The listing builds one solid part. Answer for the finished solid, in the listing's coordinates (mm). A direction names the side the tool comes from. Give positions to 0.01 mm unless a question says otherwise; leave off trailing zeros. Write each loop counter-clockwise with the first axis right and the second up, starting at its lowest first coordinate (ties: lowest second). Pieces come first, ordered by that corner, then holes.
```python
from build123d import *

# Parameters (mm, degrees)
BOSS_EXTRUDE1_DEPTH = 57
SKETCH3_R           = 47.5
SKETCH3_R_2         = 31
BOSS_EXTRUDE3_DEPTH = 13
SKETCH4_R           = 47.5
SKETCH4_R_2         = 32.5
BOSS_EXTRUDE4_DEPTH = 37
SKETCH5_R           = 47.5
SKETCH5_R_2         = 31
BOSS_EXTRUDE5_DEPTH = 11
SKETCH8_R           = 19
BOSS_EXTRUDE6_DEPTH = 3
SKETCH9_W           = 85.5
SKETCH9_H           = 94
CUT_EXTRUDE1_DEPTH  = 3
CUT_EXTRUDE3_DEPTH  = 29.5
CUT_EXTRUDE4_DEPTH  = 36


with BuildPart() as part:
    # Sketch1 → Boss-Extrude1 (new body, symmetric)
    with BuildSketch(Plane(origin=(0, 0, 0), x_dir=(1, 0, 0), z_dir=(0, 1, 0))):
        Polygon((-102, 0), (-97, 16), (97, 16), (102, 0), (0, 0), align=None)
    extrude(amount=BOSS_EXTRUDE1_DEPTH, both=True)

    # Sketch3 → Boss-Extrude3 (add)
    with BuildSketch(Plane(origin=(0, 0, -16), x_dir=(-1, 0, 0), z_dir=(0, 0, -1))):
        with Locations(Location((0, 0, 0), (0, 0, 180))):  # turned: the seam where the file's is
            Circle(SKETCH3_R)
        Circle(SKETCH3_R_2, mode=Mode.SUBTRACT)
    extrude(amount=BOSS_EXTRUDE3_DEPTH)

    # Sketch4 → Boss-Extrude4 (add)
    with BuildSketch(Plane(origin=(0, 0, -29), x_dir=(-1, 0, 0), z_dir=(0, 0, -1))):
        with Locations(Location((0, 0, 0), (0, 0, 180))):  # turned: the seam where the file's is
            Circle(SKETCH4_R)
        Circle(SKETCH4_R_2, mode=Mode.SUBTRACT)
    extrude(amount=BOSS_EXTRUDE4_DEPTH)

    # Sketch5 → Boss-Extrude5 (add)
    with BuildSketch(Plane(origin=(0, 0, -66), x_dir=(-1, 0, 0), z_dir=(0, 0, -1))):
        with Locations(Location((0, 0, 0), (0, 0, 180))):  # turned: the seam where the file's is
            Circle(SKETCH5_R)
        Circle(SKETCH5_R_2, mode=Mode.SUBTRACT)
    extrude(amount=BOSS_EXTRUDE5_DEPTH)

    # Sketch8 → Boss-Extrude6 (add)
    with BuildSketch(Plane(origin=(0, 0, -16), x_dir=(-1, 0, 0), z_dir=(0, 0, -1))):
        with Locations(Location((-70, 28, 0), (0, 0, 180))):  # turned: the seam where the file's is
            Circle(SKETCH8_R)
        with Locations(Location((-70, -28, 0), (0, 0, 180))):  # turned: the seam where the file's is
            Circle(SKETCH8_R)
    boss_extrude6 = extrude(amount=BOSS_EXTRUDE6_DEPTH)

    # Sketch9 → Cut-Extrude1 (cut)
    with BuildSketch(Plane.XY):
        with Locations((49.25, 0)):
            Rectangle(SKETCH9_W, SKETCH9_H)
    cut_extrude1 = extrude(amount=-CUT_EXTRUDE1_DEPTH, mode=Mode.SUBTRACT)

    # Sketch6 → Cut-Extrude3 (cut, symmetric)
    with BuildSketch(Plane(origin=(0, 0, -16), x_dir=(-1, 0, 0), z_dir=(0, 0, -1))):
        with BuildLine():
            Line((-73, 36), (-67, 36))
            ThreePointArc((-67, 36), (-59, 28), (-67, 20))
            Line((-67, 20), (-73, 20))
            ThreePointArc((-73, 20), (-81, 28), (-73, 36))
        make_face()
    cut_extrude3 = extrude(amount=CUT_EXTRUDE3_DEPTH, both=True, mode=Mode.SUBTRACT)

    # Sketch7 → Cut-Extrude4 (cut, symmetric)
    with BuildSketch(Plane(origin=(0, 0, -16), x_dir=(-1, 0, 0), z_dir=(0, 0, -1))):
        with BuildLine():
            Line((-73, -20), (-67, -20))
            ThreePointArc((-67, -20), (-59, -28), (-67, -36))
            Line((-67, -36), (-73, -36))
            ThreePointArc((-73, -36), (-81, -28), (-73, -20))
        make_face()
    cut_extrude4 = extrude(amount=CUT_EXTRUDE4_DEPTH, both=True, mode=Mode.SUBTRACT)

    # Mirror1: Boss-Extrude6, Cut-Extrude1, Cut-Extrude3, Cut-Extrude4 across plane
    add(boss_extrude6.mirror(Plane(origin=(0, 0, 0), x_dir=(0, 0, 1), z_dir=(1, 0, 0))))
    add(cut_extrude1.mirror(Plane(origin=(0, 0, 0), x_dir=(0, 0, 1), z_dir=(1, 0, 0))), mode=Mode.SUBTRACT)
    add(cut_extrude3.mirror(Plane(origin=(0, 0, 0), x_dir=(0, 0, 1), z_dir=(1, 0, 0))), mode=Mode.SUBTRACT)
    add(cut_extrude4.mirror(Plane(origin=(0, 0, 0), x_dir=(0, 0, 1), z_dir=(1, 0, 0))), mode=Mode.SUBTRACT)


solid = part.part
```
Item 1: Which of the six approach directions +Z, -Z, +X, -X, +Y, -Y give full straight-line access (tool end or side, diameter ignored) to faces 1 (the face through (-31, 9.76, -47.24)), 2 (the face through (51.02, 27.16, -17.48)), 3 (the face through (-69.7, 36.2, -19)), 4 (the face through (70, -36, -11))?
Conclusion:
face 1: none
face 2: -Z
face 3: -Z, -X, +Y, -Y
face 4: +Z, -Z
Item 2: Determine the mould class of faces 5 (the face through (31, 10, -77)), 6 (the face through (99.465, 0.798, -8.112)), 7 (the face through (-70, 36, -11)) for opening direction X: pulls with the +X half, pulls with the -X half, needs draft (parallel to the pull), parting line crosses it, or undercut.
Conclusion:
face 5: needs draft
face 6: pulls with the +X half
face 7: undercut
Item 3: Consider probe 1 along Y at (x, z) = (0, -71); probe 2 along Y at (x, z) = (0, -53); probe 3 along Z at (x, y) = (-58.5, 8). Determine where each line is inside the solid, lowest interval first.
Conclusion:
probe 1: y = -47.5 to -31, 31 to 47.5
probe 2: y = -47.5 to -32.5, 32.5 to 47.5
probe 3: z = -16 to -3
Item 4: A cutting plane is placed at C-C, the plane z = -26.5. Give the vertices of the cut face in (x, y), plus the area to 3 significant figures.
Conclusion:
outline: circle Ø95 at (0, 0); hole circle Ø62 at (0, 0)
area: 4,070 mm2
Item 5: A cutting plane is placed at A-A, the plane x = -70. Give the vertices of the cut face in (y, z).
Conclusion:
outline: (-57, -16) - (-47, -16) - (-47, -19) - (-36, -19) - (-36, -3) - (-47, -3) - (-47, 0) - (-57, 0) - close; (-20, -19) - (-9, -19) - (-9, -16) - (9, -16) - (9, -19) - (20, -19) - (20, -3) - (-20, -3) - close; (36, -19) - (47, -19) - (47, -16) - (57, -16) - (57, 0) - (47, 0) - (47, -3) - (36, -3) - close
Item 6: A cutting plane is placed at D-D, the plane y = -40.5. Give the vertices of the cut face in (x, z), plus the area to 3 significant figures.
Conclusion:
outline: (-102, 0) - (-97, -16) - (-84.31, -16) - (-84.31, -19) - (-55.69, -19) - (-55.69, -16) - (-24.82, -16) - (-24.82, -77) - (24.82, -77) - (24.82, -16) - (55.69, -16) - (55.69, -19) - (84.31, -19) - (84.31, -16) - (97, -16) - (102, 0) - (92, 0) - (92, -3) - (6.5, -3) - (6.5, 0) - (-6.5, 0) - (-6.5, -3) - (-92, -3) - (-92, 0) - close
area: 5,870 mm2
Item 7: A cutting plane is placed at B-B, the plane x = 0. Give the vertices of the cut face in (y, z).
Conclusion:
outline: (-57, -16) - (-47.5, -16) - (-47.5, -77) - (-31, -77) - (-31, -66) - (-32.5, -66) - (-32.5, -29) - (-31, -29) - (-31, -16) - (31, -16) - (31, -29) - (32.5, -29) - (32.5, -66) - (31, -66) - (31, -77) - (47.5, -77) - (47.5, -16) - (57, -16) - (57, 0) - (-57, 0) - close
Item 8: Each of these flat-tipped pins is pushed along its axis until it touches: P1, Ø4, axis at x = 76.5, y = 10.5, coming from the +Z side; P2, Ø0.9, axis at y = -0.5, z = -1.5, coming from the -X side; P3, Ø8, axis at x = -40.5, y = 42.5, coming from the -Z side; P4, Ø3.5, axis at y = -20.5, z = -1.5, coming from the +X side. Where does it stop, or does it pass through?
Conclusion:
P1: stops at z = -3
P2: stops at x = -101.67
P3: stops at z = -16
P4: stops at x = 102
